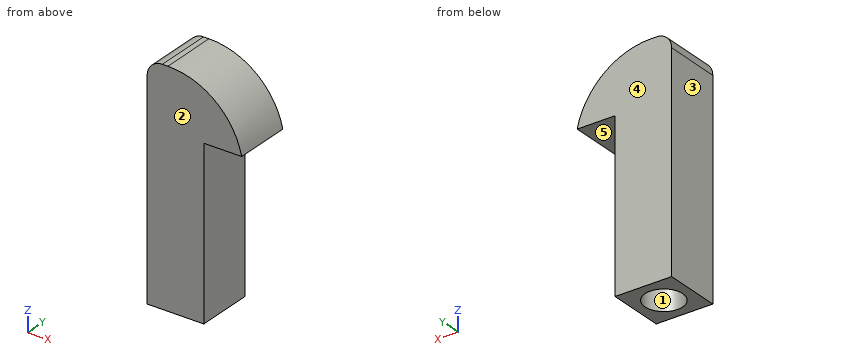
```python
from build123d import *

# Parameters (mm, degrees)
SKETCH1_W                         = 9.525
SKETCH1_H                         = 9.525
EXTRUDE1_DEPTH                    = 38.1
F_1_4_20_TAPPED_HOLE1_D           = 5.1054
F_1_4_20_TAPPED_HOLE1_DEPTH       = 21.336
F_1_4_20_TAPPED_HOLE1_CBORE_D     = 6.35
F_1_4_20_TAPPED_HOLE1_CBORE_DEPTH = 14.986
F_1_4_20_TAPPED_HOLE1_TIP         = 1.533816902
SKETCH9_W                         = 10
SKETCH9_H                         = 9.525
EXTRUDE3_DEPTH                    = 6.35
FILLET2_R                         = 12.7
FILLET3_R                         = 2.54


with BuildPart() as part:
    # Sketch1 → Extrude1 (new body)
    with BuildSketch(Plane.XY):
        with Locations((-4.7625, 4.7625)):
            Rectangle(SKETCH1_W, SKETCH1_H)
    extrude(amount=EXTRUDE1_DEPTH)

    # 1/4-20 Tapped Hole1
    with Locations(Plane(origin=(-4.7625, 4.7625, 0), x_dir=(-1, 0, 0), z_dir=(0, 0, -1))):
        with Locations((0, 0)):
            CounterBoreHole(F_1_4_20_TAPPED_HOLE1_D / 2, F_1_4_20_TAPPED_HOLE1_CBORE_D / 2, F_1_4_20_TAPPED_HOLE1_CBORE_DEPTH, depth=F_1_4_20_TAPPED_HOLE1_DEPTH)
            with Locations((0, 0, -(F_1_4_20_TAPPED_HOLE1_DEPTH + F_1_4_20_TAPPED_HOLE1_TIP / 2))):  # 118° drill point
                Cone(0, F_1_4_20_TAPPED_HOLE1_D / 2, F_1_4_20_TAPPED_HOLE1_TIP, mode=Mode.SUBTRACT)

    # Sketch9 → Extrude3 (add)
    with BuildSketch(Plane(origin=(0, 0, 0), x_dir=(0, 0, -1), z_dir=(1, 0, 0))):
        with Locations((-33.1, 4.7625)):
            Rectangle(SKETCH9_W, SKETCH9_H)
    extrude(amount=EXTRUDE3_DEPTH)

    # Fillet2
    # the kernel refuses this fillet: 12.7 mm, written as the material it takes off along each edge
    with BuildSketch(Plane(origin=(6.35, -31.024184115, 38.1), x_dir=(-1, 0, 0), z_dir=(0, 1, 0))) as fillet2_piece_1:
        with BuildLine():
            CenterArc((12.409673646, -12.7), FILLET2_R, 90, 77.725329785)
            Line((0, -10), (-0.248193473, -9.946))
            ThreePointArc((-0.248193473, -9.946), (-0.254, -5), (-0.254, 0))
            Line((-0.254, 0), (0, 0.254))
            Line((0, 0.254), (12.409673646, 0.254))
            Line((12.409673646, 0.254), (12.409673646, 0))
        make_face()
    extrude(amount=71.57336823, mode=Mode.SUBTRACT)

    # Fillet3
    fillet3_edges = [part.edges().sort_by_distance(p)[0] for p in [
        (-9.525, 4.7625, 38.1),
    ]]
    fillet(fillet3_edges, radius=FILLET3_R)


solid = part.part
```
Read the model definition and answer for the solid it produces. Units are mm, in the model's axes. Face numbers are marked on the shaded views. A direction names the side the tool comes from. Round coordinates to 2 decimals unless told otherwise and drop trailing zeros. Write each loop counter-clockwise with the first axis right and the second up, starting at its lowest first coordinate (ties: lowest second). Pieces come first, ordered by that corner, then holes. Notation, with made-up numbers: (-17, 49.25) - (11, 49.25) arc R9 ccw to (11, 56.25) - close; hole circle Ø3 at (48, -40). An arc over 180 degrees is marked (long way). One line per item, written item: value.
Q1. Find section D-D (x = 1). Determine the outline of the cut face in (y, z) (3 decimals), and give its area (3 significant figures).
The answers:
outline: (0, 28.1) - (9.525, 28.1) - (9.525, 35.957) - (0, 35.957) - close
area: 74.8 mm2
Q2. Each of these flat-tipped pins is pushed along its axis until it touches: P1, Ø4, axis at x = -5, y = 8, coming from the -Z side; P2, Ø3, axis at x = 4.5, y = 3, coming from the -Z side; P3, Ø3, axis at x = 3.5, y = 1.5, coming from the +Z side; P4, Ø3, axis at x = -4.76, y = 4.76, coming from the -Z side. Where does it stop, or does it pass through?
The answers:
P1: stops at z = 0
P2: stops at z = 28.1
P3: stops at z = 35.21
P4: stops at z = 21.97
Q3. Which of the six approach directions +Z, -Z, +X, -X, +Y, -Y give full straight-line access (tool end or side, diameter ignored) to the marked faces 4 and 5?
The answers:
face 4: +Z, -Z, +X, -X, +Y
face 5: -Z, +X, +Y, -Y
Q4. Find section A-A (y = 8.5). Determine the outline of the cut face in (x, z) (3 decimals), and give its area (3 significant figures).
The answers:
outline: (-9.525, 0) - (0, 0) - (0, 28.1) - (6.35, 28.1) arc R12.7 ccw to (-6.06, 38.1) - (-6.985, 38.1) arc R2.54 ccw to (-9.525, 35.56) - close
area: 394 mm2
Q5. Find section C-C (z = 19.5). Determine the outline of the cut face in (x, y) (1 decimal), and give its area (3 significant figures).
The answers:
outline: (-9.5, 0) - (0, 0) - (0, 9.5) - (-9.5, 9.5) - close; hole circle Ø5.1 at (-4.8, 4.8)
area: 70.3 mm2
Q6. Find section B-B (z = 26). Determine the outline of the cut face in (x, y) (3 decimals).
The answers:
outline: (-9.525, 0) - (0, 0) - (0, 9.525) - (-9.525, 9.525) - close
Q7. For a pull along X with two mould halves and no side action, classify the marked faces 1, 2 and 3 as pulls with the +X half, pulls with the -X half, needs draft (parallel to the pull), parting line crosses it, or undercut.
The answers:
face 1: undercut
face 2: needs draft
face 3: pulls with the -X half
Q8. Straight lines are drawn through the part: line 1 (X direction, y = 2.25, z = 24) (3 decimals); line 2 (X direction, y = 6.75, z = 15.5) (3 decimals); line 3 (X direction, y = 6.25, z = 4) (3 decimals). For each, find the intervals that lie inside material, in ascending order. Write a range as from..to.
The answers:
line 1: x = -9.525..0
line 2: x = -9.525..-6.364, -3.161..0
line 3: x = -9.525..-7.567, -1.958..0
